from build123d import *

# Parameters (mm, degrees)
ESQUISSE1_W        = 30.5
ESQUISSE1_H        = 15
ESQUISSE1_R        = 2.125
BOSS_EXTRU_3_DEPTH = 2
BOSS_EXTRU_4_DEPTH = 8
CONG_3_R           = 1
CHANFREIN2_SIZE    = 1
CHANFREIN3_SIZE    = 0.5


with BuildPart() as part:
    # Esquisse1 → Boss.-Extru.3 (new body)
    with BuildSketch(Plane.XY):
        with Locations((15.25, 7.5)):
            Rectangle(ESQUISSE1_W, ESQUISSE1_H)
        with Locations((5, 7.5)):
            Circle(ESQUISSE1_R, mode=Mode.SUBTRACT)
        with Locations((25.5, 7.5)):
            Circle(ESQUISSE1_R, mode=Mode.SUBTRACT)
    extrude(amount=BOSS_EXTRU_3_DEPTH)

    # Esquisse1<5> → Boss.-Extru.4 (add)
    with BuildSketch(Plane.XY):
        with BuildLine():
            Line((12, 7.5), (12, 11.75))
            Line((12, 11.75), (10, 11.75))
            Line((10, 11.75), (10, 7.5))
            ThreePointArc((10, 7.5), (15.25, 2.25), (20.5, 7.5))
            Line((20.5, 7.5), (20.5, 11.75))
            Line((20.5, 11.75), (18.5, 11.75))
            Line((18.5, 11.75), (18.5, 7.5))
            ThreePointArc((18.5, 7.5), (15.25, 4.25), (12, 7.5))
        make_face()
    extrude(amount=-BOSS_EXTRU_4_DEPTH)

    # Congé3
    cong_3_edges = [part.edges().sort_by_distance(p)[0] for p in [
        (10, 9.625, 0),
        (10, 11.75, -4),
        (19.5, 11.75, 0),
        (20.5, 9.625, -8),
        (20.5, 11.75, -4),
        (15.25, 2.25, -8),
        (10, 9.625, -8),
        (15.25, 2.25, 0),
        (20.5, 9.625, 0),
        (11, 11.75, 0),
    ]]
    fillet(cong_3_edges, radius=CONG_3_R)

    # Chanfrein2
    chanfrein2_edges = [part.edges().sort_by_distance(p)[0] for p in [
        (23.375, 7.5, 0),
        (2.875, 7.5, 0),
    ]]
    chamfer(chanfrein2_edges, length=CHANFREIN2_SIZE)

    # Chanfrein3
    chanfrein3_edges = [part.edges().sort_by_distance(p)[0] for p in [
        (0, 0, 1),
        (0, 15, 1),
        (0, 7.5, 2),
        (0, 7.5, 0),
        (15.25, 15, 0),
        (30.5, 7.5, 0),
        (15.25, 0, 0),
    ]]
    chamfer(chanfrein3_edges, length=CHANFREIN3_SIZE)


solid = part.part
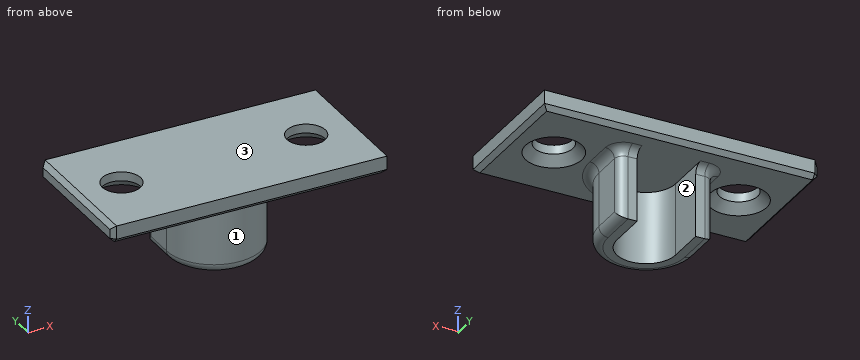
Design review of the part built by this model. Coordinates are the model's own, in mm. Face numbers are marked on the shaded views. Give positions to 0.01 mm unless a question says otherwise; leave off trailing zeros. Order: outer loops, then holes, each group sorted by start corner. A loop starts at its lowest first (then second) coordinate and runs counter-clockwise, first axis right, second up. Notation, with made-up numbers: (39.25, 42) - (79.25, 42) arc R10 cw to (79.25, 47) - close; hole circle Ø10 at (-4.5, 14). An arc over 180 degrees is marked (long way). Use CSV: the item, a comma, the result in double quotes. Start each with the question number.
Q1. For P1, Ø1, axis at y = 9.5, z = -5.5, coming from the -X side; P2, Ø0.8, axis at x = 19, z = -4, coming from the +Y side; P3, Ø1, axis at x = 20, z = -5.5, coming from the -Y side, all flat-tipped, find the tip position at first contact; note any pin that passes through.
Q2. Take a section at C-C (x = 15.25). State the section outline as (y, z) points, and give its area (4 significant figures).
Q3. For line 1 (Y direction, x = 5, z = 1.4) (3 decimals); line 2 (X direction, y = 8, z = -3.75); line 3 (Z direction, x = 5, y = 1.25), list the stretches that pass through material, from the lowest coordinate up.
Q4. Take a section at A-A (x = 5). State the section outline as (y, z) points (3 decimals), and give its area (4 significant figures).
Q5. Take a section at B-B (z = -5.5). State the section outline as (x, y) points, and give its area (3 significant figures).
Q6. Draft analysis for pull direction X (two halves, no side actions). For the marked faces 1, 2 and 3, state which applies: pulls with the +X half, pulls with the -X half, needs draft (parallel to the pull), parting line crosses it, or undercut.
Calculated:
1,P1,"stops at x = 10"
1,P2,"stops at y = 11.75"
1,P3,"stops at y = 4.42"
2,outline,"(0, 0.5) - (0.5, 0) - (1.25, 0) arc R1 cw to (2.25, -1) - (2.25, -7) arc R1 ccw to (3.25, -8) - (4.25, -8) - (4.25, 0) - (14.5, 0) - (15, 0.5) - (15, 2) - (0, 2) - close"
2,area,"45.75 mm²"
3,line 1,"y = 0 to 5.375, 9.625 to 15"
3,line 2,"x = 10 to 12, 18.5 to 20.5"
3,line 3,"z = 0 to 2"
4,outline,"(0, 0.5) - (0.5, 0) - (4.375, 0) - (5.375, 1) - (5.375, 2) - (0, 2) - close; (9.625, 1) - (10.625, 0) - (14.5, 0) - (15, 0.5) - (15, 2) - (9.625, 2) - close"
4,area,"20.25 mm²"
5,outline,"(10, 7.5) arc R5.25 ccw to (20.5, 7.5) - (20.5, 10.75) arc R1 ccw to (19.5, 11.75) - (18.5, 11.75) - (18.5, 7.5) arc R3.25 cw to (12, 7.5) - (12, 11.75) - (11, 11.75) arc R1 ccw to (10, 10.75) - close"
5,area,"43.3 mm²"
6,face 1,"parting line crosses it"
6,face 2,"undercut"
6,face 3,"needs draft"
